Source: CAD feature listing. Evaluate the final solid. Frame: model axes, mm. A direction names the side the tool comes from. Give positions to 0.01 mm unless a question says otherwise; leave off trailing zeros. Loops run counter-clockwise (first coordinate to the right, second up) from the corner with the lowest first, then second, coordinate; pieces in that order, holes last. Notation, with made-up numbers: M 57.5,13.5 L 77.5,13.5 A21 cw 77.5,25.5 Z; hole C 8.5,-28 d2. An arc over 180 degrees is marked long. Write item = value, one per line.
from build123d import *

# Parameters (mm, degrees)
F0_W     = 117.475
F0_H     = 12.7
F1_DEPTH = 63.5
F2_W     = 117.475
F2_H     = 40.322089
F3_DEPTH = 12.7
F4_W     = 60.325
F4_H     = 40.322089
F5_DEPTH = 22.225
F6_R     = 9.525
F7_DEPTH = 25.4
F8_R     = 10.010488
F9_DEPTH = 47.879


with BuildPart() as f1:
    # F0 (on Front) → F1 (new body)
    with BuildSketch(Plane.XZ):
        with Locations((4.799338, -20.741718)):
            Rectangle(F0_W, F0_H)
    extrude(amount=F1_DEPTH)

    # F2 (on face) → F3 (join)
    with BuildSketch(Plane.XY.offset(-14.391718)):
        with Locations((4.799338, -30.519849)):
            Rectangle(F2_W, F2_H)
    extrude(amount=F3_DEPTH)

    # F4 (on face) → F5 (join)
    with BuildSketch(Plane.XY.offset(-1.691718)):
        with Locations((-23.775662, -30.519849)):
            Rectangle(F4_W, F4_H)
    extrude(amount=F5_DEPTH)

    # F6 (on face) → F7 (cut)
    with BuildSketch(Plane.XY.offset(-1.691718)):
        with Locations((31.786838, -28.455894)):
            Circle(F6_R)
    extrude(amount=-F7_DEPTH, mode=Mode.SUBTRACT)

    # F8 (on face) → F9 (cut)
    with BuildSketch(Plane.XY.offset(20.533282)):
        with Locations((-23.775662, -28.455894)):
            Circle(F8_R)
    extrude(amount=-F9_DEPTH, mode=Mode.SUBTRACT)


solid = f1.part
1. Material intervals for probe 1 along Y at (x, z) = (13, -10); probe 2 along X at (y, z) = (-20, 14.5); probe 3 along Z at (x, y) = (-8, -60.5), sorted ascending. Write a range as from..to.
Derived:
probe_1 = -50.68..-10.36
probe_2 = -53.94..-29.13, -18.42..6.39
probe_3 = -27.09..-14.39
2. Pull-direction query (Y, two-part tool) for faces 5 (the cylindrical face through (40.87, -25.59, -14.21)), 6 (the flat face through (4, -63.5, -21)), 7 (the flat face through (6.387, -31, 9)); classes: +Y half, -Y half, draft (parallel to the pull), parting line (faces both ways), or undercut.
Derived:
face_5 = undercut
face_6 = -Y half
face_7 = draft
3. Cut plane A-A, the plane x = -15.5. Return the cut outline in (y, z).
Derived:
outline = M -63.5,-27.09 L -34.09,-27.09 L -34.09,20.53 L -50.68,20.53 L -50.68,-14.39 L -63.5,-14.39 Z; M -22.82,-27.09 L 0,-27.09 L 0,-14.39 L -10.36,-14.39 L -10.36,20.53 L -22.82,20.53 Z
4. Cut plane B-B, the plane y = -33. Return the cut outline in (x, z), then the cut area to 3 significant figures.
Derived:
outline = M -53.94,-27.09 L -32.7,-27.09 L -32.7,20.53 L -53.94,20.53 Z; M -14.86,-27.09 L 23.42,-27.09 L 23.42,-1.69 L 6.39,-1.69 L 6.39,20.53 L -14.86,20.53 Z; M 40.16,-27.09 L 63.54,-27.09 L 63.54,-1.69 L 40.16,-1.69 Z
area = 3,050 mm²
5. Cut plane D-D, the plane z = 2. Return the cut outline in (x, y).
Derived:
outline = M -53.94,-50.68 L 6.39,-50.68 L 6.39,-10.36 L -53.94,-10.36 Z; hole C -23.78,-28.46 d20.02
6. Reachability of faces 1 (the flat face through (4, -57, -14.392)), 2 (the flat face through (-53.938, -32, -4)), 3 (the flat face through (41, -35, -1.692)), 4 (the flat face through (4, -5, -14.392)) from +Z, -Z, +X, -X, +Y, -Y: full face, straight path, thin tool, end or side. Return the list, or none.
Derived:
face_1 = +Z, +X, -X, -Y
face_2 = +Z, -Z, -X, +Y, -Y
face_3 = +Z, +X, +Y, -Y
face_4 = +Z, +X, -X, +Y
7. First-contact query: pin 1 Ø8 at (x, y) = (13, -53) entering from +Z; pin 2 Ø4 at (x, z) = (-6, 4.5) entering from +Y; pin 3 Ø5 at (x, y) = (2.5, -6.5) entering from +Z; pin 4 Ø10.5 at (x, y) = (-10.5, -55) entering from +Z. Flat tips, straight axial feed; report the tip coordinate or a pass-through.
Derived:
pin_1 = -1.69
pin_2 = -10.36
pin_3 = -14.39
pin_4 = 20.53
8. Cut plane C-C, the plane x = 51. Return the cut outline in (y, z), then the cut area to 3 significant figures.
Derived:
outline = M -63.5,-27.09 L 0,-27.09 L 0,-14.39 L -10.36,-14.39 L -10.36,-1.69 L -50.68,-1.69 L -50.68,-14.39 L -63.5,-14.39 Z
area = 1,320 mm²
